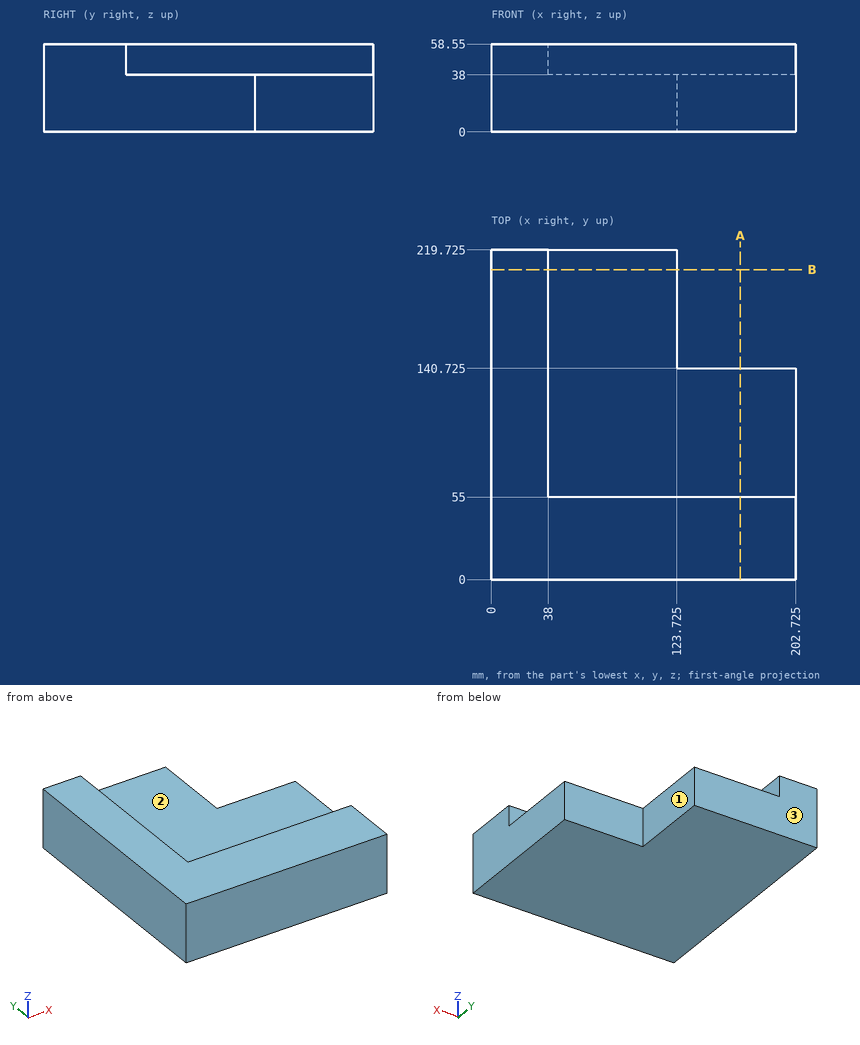
Job drawing, mm, ordinate dimensions from the low corner. One solid piece. A direction names the side the tool comes from. Coordinates: 2 decimals unless noted, no trailing zeros. Loops run counter-clockwise (first coordinate to the right, second up) from the corner with the lowest first, then second, coordinate; pieces in that order, holes last. Notation, with made-up numbers: (32, 78.5) - (79, 78.5) arc R5 cw to (79, 87.5) - close; hole circle Ø7 at (-37, 83). An arc over 180 degrees is marked (long way). Write item = value, one per line. Start each with the question number.
Q1. Cut at A-A, the plane x = 166. List the corners of the cut face in (y, z) (3 decimals), then the cut area to 3 significant figures.
Q2. Flat gauge pins, fed straight in: pin 1 Ø4 at (x, y) = (56, 104.5) entering from +Z; pin 2 Ø4 at (y, z) = (143, 40.5) entering from +X; pin 3 Ø3 at (x, z) = (152.5, 22) entering from +Y (3 decimals). Where does each tip first touch, or does it go through?
Q3. Which spindle directions (+Z, -Z, +X, -X, +Y, -Y) get a long thin tool onto all of the face, cutting with end or side? Do the marked faces 1, 2 and 3. Say none if no direction does.
Q4. Drill centre lines: L1, parallel to X at y = 188.5, z = 55; L2, parallel to Y at x = 125, z = 11 (3 decimals). Where is each one in solid material? Low to high.
Q5. Cut at B-B, the plane y = 206.5. List the corners of the cut face in (x, z) (3 decimals), then the cut area to 3 significant figures.
Computed:
q1.outline = (0, 0) - (140.725, 0) - (140.725, 38) - (55, 38) - (55, 58.55) - (0, 58.55) - close
q1.area = 6,480 mm²
q2.pin_1 = 38
q2.pin_2 = 38
q2.pin_3 = 140.725
q3.face_1 = +Z, -Z, +X, +Y
q3.face_2 = +Z, +X, +Y
q3.face_3 = +Z, -Z, +X, -X, +Y
q4.L1 = 0 to 38
q4.L2 = 0 to 140.725
q5.outline = (0, 0) - (123.725, 0) - (123.725, 38) - (38, 38) - (38, 58.55) - (0, 58.55) - close
q5.area = 5,480 mm²
